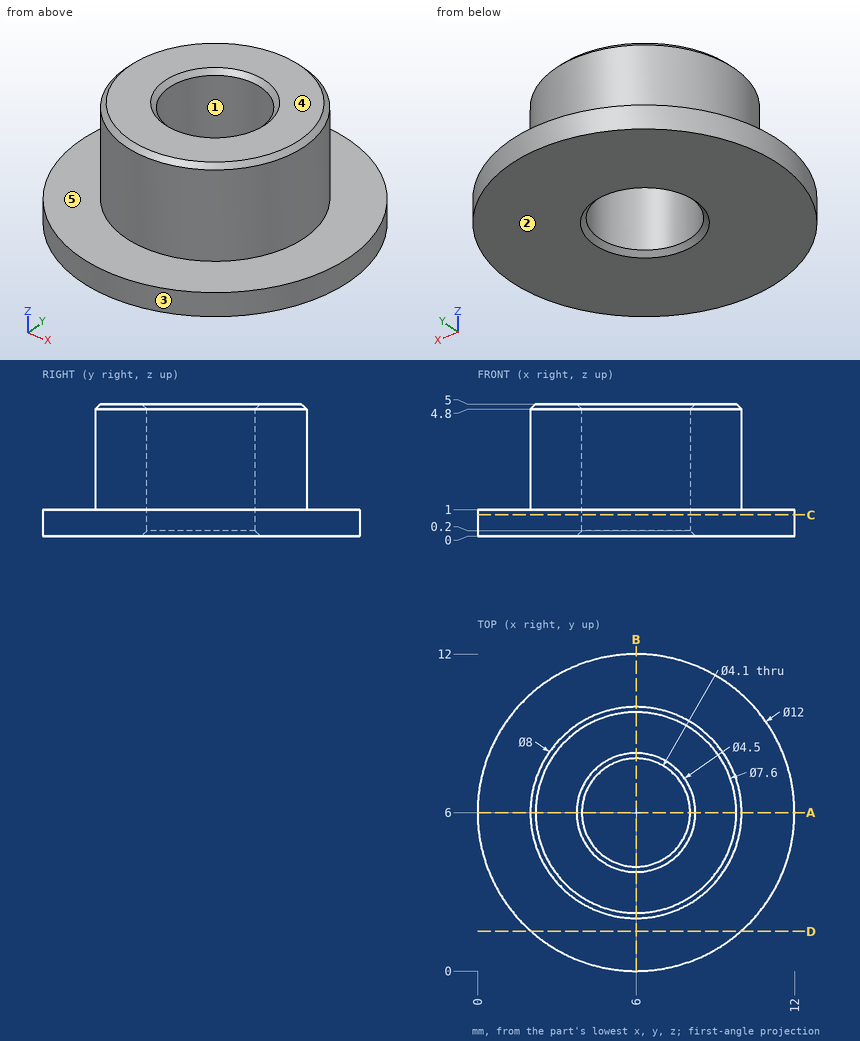
Here's the drawing with two shaded views (mm, measured from the low corner). I have some questions. A direction names the side the tool comes from. Give positions to 0.01 mm unless a question says otherwise; leave off trailing zeros. Loops run counter-clockwise (first coordinate to the right, second up) from the corner with the lowest first, then second, coordinate; pieces in that order, holes last. Notation, with made-up numbers: M 43.5,81.5 L 52.5,81.5 A14 ccw 52.5,107.5 Z; hole C 46,-36.5 d9. An arc over 180 degrees is marked long. Answer in a Markdown table with one row per item.
1. For pin 1 Ø2 at (x, z) = (7.5, 2.5) entering from +Y; pin 2 Ø1 at (x, z) = (9, 3.5) entering from +Y; pin 3 Ø1 at (y, z) = (9.5, 2.5) entering from -X, each with a flat end and sliding along its axis, tell me the tip position at first contact or that it passes through.
Taken from the geometry:
| item | result |
|---|---|
| pin 1 | stops at y = 9.97 |
| pin 2 | stops at y = 9.12 |
| pin 3 | stops at x = 3.35 |
2. Thinking about a two-plate mould opening in X: for the marked faces 1, 2 and 3, which applies, released by +X, released by -X, zero draft, split by the parting line, or undercut?
Taken from the geometry:
| item | result |
|---|---|
| face 1 | undercut |
| face 2 | zero draft |
| face 3 | split by the parting line |
3. If I drill on line 1 along Y through (x, z) = (6, 4.7); line 2 along Z through (x, y) = (4, 10.75); line 3 along Y through (x, z) = (7.25, 4.1), over which ranges is the centre line in solid material (lowest first)?
Taken from the geometry:
| item | result |
|---|---|
| line 1 | y = 2 to 3.95, 8.05 to 10 |
| line 2 | z = 0 to 1 |
| line 3 | y = 2.2 to 4.38, 7.62 to 9.8 |
4. Suppose I cut it at A-A on y = 6. Write out the boundary of the cut face in (x, z).
Taken from the geometry:
| item | result |
|---|---|
| outline | M 0,0 L 3.75,0 L 3.95,0.2 L 3.95,4.8 L 3.75,5 L 2.2,5 L 2,4.8 L 2,1 L 0,1 Z; M 8.05,0.2 L 8.25,0 L 12,0 L 12,1 L 10,1 L 10,4.8 L 9.8,5 L 8.25,5 L 8.05,4.8 Z |
5. Which directions (+Z, -Z, +X, -X, +Y, -Y) give clear straight access to the entire face, cutting with the end or side of a thin tool? Please do the marked faces 4 and 5.
Taken from the geometry:
| item | result |
|---|---|
| face 4 | +Z, +X, -X, +Y, -Y |
| face 5 | +Z |
6. Suppose I cut it at D-D on y = 1.5. Write out the boundary of the cut face in (x, z).
Taken from the geometry:
| item | result |
|---|---|
| outline | M 2.03,0 L 9.97,0 L 9.97,1 L 2.03,1 Z |
7. Suppose I cut it at C-C on z = 0.8. Write out the boundary of the cut face in (x, y).
Taken from the geometry:
| item | result |
|---|---|
| outline | C 6,6 d12; hole C 6,6 d4.1 |
